Geometry check sheet. Reference: the model listing, model coordinates, mm. Face numbers are marked on the shaded views. Give positions to 0.01 mm unless a question says otherwise; leave off trailing zeros. Write each loop counter-clockwise with the first axis right and the second up, starting at its lowest first coordinate (ties: lowest second). Pieces come first, ordered by that corner, then holes. Notation, with made-up numbers: (16.25, 4) - (60.25, 4) arc R20 cw to (60.25, 22) - close; hole circle Ø5 at (33.25, -26). An arc over 180 degrees is marked (long way). Write item = value, one per line. Start each with the question number.
(1) Depth check by flat-ended pin: pin 1 Ø8 at (x, z) = (54.5, -41) entering from -Y; pin 2 Ø2 at (y, z) = (-160, -88.5) entering from +X; pin 3 Ø10 at (x, y) = (12, -145) entering from +Z. Enter the tip coordinate at first touch or a pass-through.
(2) Section check A-A, the plane y = -237. Enter the section's corners in (x, z).
(3) Section check B-B, the plane x = 21.5. Enter the section's corners in (y, z).
(4) Draft check along Z on the marked faces 1 and 2. Enter one of: pulls with the +Z half, pulls with the -Z half, needs draft (parallel to the pull), parting line crosses it, or undercut.
(5) Section check C-C, the plane z = -199. Enter the section's corners in (x, y) (1 decimal).
(6) Thickness scan on L1, parallel to Z at x = 2.5, y = -110; L2, parallel to Y at x = 78, z = 253.5; L3, parallel to X at y = -99, z = 274. Record the ranges inside material, lowest first.
```python
from build123d import *

# Parameters (mm, degrees)
EXTRUDE_THIN1_DEPTH      = 342.9
BOSS_EXTRUDE3_REACH      = 442.49
BOSS_EXTRUDE3_END_RADIUS = 411.1625
SKETCH8_R                = 19.05


with BuildPart() as part:
    # Sketch1 → Extrude-Thin1 (new, symmetric)
    with BuildSketch(Plane.XY):
        with BuildLine():
            ThreePointArc((0, 0), (28.7854342, -135.80582632), (101.6, -254))
            Line((101.6, -254), (98.031425453, -257.153836069))
            ThreePointArc((98.031425453, -257.153836069), (24.36356396, -137.574574416), (-4.759199547, -0.177273569))
            Line((-4.759199547, -0.177273569), (0, 0))
        make_face()
    extrude(amount=EXTRUDE_THIN1_DEPTH, both=True)

    # Boss-Extrude3: up to this cylinder (the profile starts outside it)
    boss_extrude3_end = Plane(origin=(406.118361376, 15.12734455, 0), z_dir=(0, 0, -1)) * Cylinder(BOSS_EXTRUDE3_END_RADIUS, 2089.305, mode=Mode.PRIVATE)
    # Sketch8 → Boss-Extrude3 (add, up to the surface)
    with BuildSketch(Plane(origin=(0, -257.153836069, 0), x_dir=(1, 0, 0), z_dir=(0, 1, 0)), mode=Mode.PRIVATE) as boss_extrude3_sk1:
        with Locations(Location((14.290800453, -190.5, 0), (0, 0, 180.000000002))):
            Circle(SKETCH8_R)
    boss_extrude3_tool1 = extrude(boss_extrude3_sk1.sketch, amount=BOSS_EXTRUDE3_REACH, mode=Mode.PRIVATE) - boss_extrude3_end
    add(boss_extrude3_tool1.solids().sort_by_distance((14.2908, -257.153836, 190.5))[0])
    # Sketch8 → Boss-Extrude3 (add, up to the surface)
    with BuildSketch(Plane(origin=(0, -257.153836069, 0), x_dir=(1, 0, 0), z_dir=(0, 1, 0)), mode=Mode.PRIVATE) as boss_extrude3_sk2:
        with Locations(Location((14.290800453, 190.5, 0), (0, 0, 90))):
            Circle(SKETCH8_R)
    boss_extrude3_tool2 = extrude(boss_extrude3_sk2.sketch, amount=BOSS_EXTRUDE3_REACH, mode=Mode.PRIVATE) - boss_extrude3_end
    add(boss_extrude3_tool2.solids().sort_by_distance((14.2908, -257.153836, -190.5))[0])


solid = part.part
```
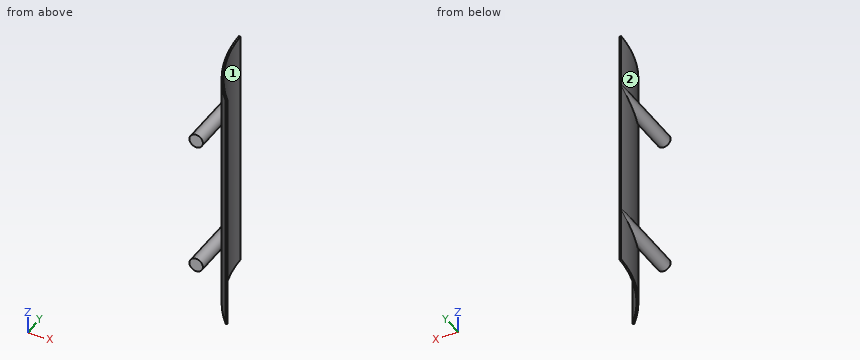
Model answer:
q1.pin_1 = -204.45
q1.pin_2 = 39.87
q1.pin_3 = 209.55
q2.outline = circle Ø38.1 at (14.29, -190.5); circle Ø38.1 at (14.29, 190.5); (81.33, -342.9) - (87.38, -342.9) - (87.38, 342.9) - (81.33, 342.9) - close
q3.outline = (-257.15, -208.13) - (-130.21, -208.13) - (-130.21, -342.9) - (-116.13, -342.9) - (-116.13, 342.9) - (-130.21, 342.9) - (-130.21, 208.13) - (-257.15, 208.13) - (-257.15, 172.87) - (-130.21, 172.87) - (-130.21, -172.87) - (-257.15, -172.87) - close
q4.face_1 = needs draft
q4.face_2 = undercut
q5.outline = (-4.8, -0.2) arc R411.2 ccw to (-2.8, -28.2) - (-2.8, -257.2) - (31.3, -257.2) - (31.3, -154) arc R411.2 ccw to (98, -257.2) - (101.6, -254) arc R406.4 cw to (0, 0) - close
q6.L1 = -205.46 to -175.54, 175.54 to 205.46
q6.L2 = -232.65 to -224.66
q6.L3 = 11.11 to 16.07
